The listing builds one solid part. Answer for the finished solid, in the listing's coordinates (mm). Face numbers are marked on the shaded views. A direction names the side the tool comes from. Round coordinates to 2 decimals unless told otherwise and drop trailing zeros. Loops run counter-clockwise (first coordinate to the right, second up) from the corner with the lowest first, then second, coordinate; pieces in that order, holes last. Notation, with made-up numbers: M 10,-25.75 L 29,-25.75 A23 ccw 29,-11.75 Z; hole C 6.5,17.5 d3. An arc over 180 degrees is marked long. Put each result on its own line as item: value. Start each with the question number.
(1) Which of the six approach directions +Z, -Z, +X, -X, +Y, -Y give full straight-line access (tool end or side, diameter ignored) to the marked faces 1, 2 and 3?
(2) Determine the mould class of the marked faces 4, 5, 6 and 7 for opening direction Z: released by +Z, released by -Z, zero draft, split by the parting line, or undercut.
(3) Section C-C, the plane y = 3.2 is taken. Determine the outline of the cut face in (x, z) (3 decimals).
(4) Straight lines are drawn through the part: line 1 (Y direction, x = -2.5, z = -3.25); line 2 (X direction, y = 1.45, z = -0.75); line 3 (Y direction, x = -1.25, z = 0.5). For each, find the intervals that lie inside material, in ascending order.
(5) Section D-D, the plane x = -2.75 is taken. Determine the outline of the cut face in (y, z), then the cut area to 3 significant figures.
(6) Flat-ended cylindrical pins translate along their axes: P1, Ø1, axis at y = 1.5, z = -2, coming from the +X side; P2, Ø1.5, axis at y = 3, z = -1, coming from the +X side; P3, Ø1.6, axis at x = -0.5, z = -0.5, coming from the -Y side. Find the tip coordinate at first contact, or state that the pin passes through.
(7) Section B-B, the plane x = -1 is taken. Determine the outline of the cut face in (y, z).
(8) Section A-A, the plane y = 0.3 is taken. Determine the outline of the cut face in (x, z) (3 decimals).
Autodesk Fusion 360 part; units mm, degrees
sketch "Sketch1" plane through (0, 0, 0) normal (0, 1, 0) x (1, 0, 0)
  line L0 (4.575, -1.7) -> (-4.575, -1.7)
  line L1 (-4.575, -1.7) -> (-4.575, 1.7)
  line L2 (-4.575, 1.7) -> (4.575, 1.7)
  line L3 (4.575, 1.7) -> (4.575, -1.7)
  line L4 (4.575, -1.7) -> (-4.575, 1.7) construction
  line L5 (-4.575, -1.7) -> (4.575, 1.7) construction
  dimension "d1" = 9.15
  dimension "d2" = 3.4
extrude "Extrude1" add sketch "Sketch1" along normal blind 4
sketch "Sketch2" plane through (0, 0, 0) normal (0, -1, 0) x (1, 0, 0)
  line L0 (-4.575, -1.7) -> (4.575, -1.7)
  line L1 (4.575, -1.7) -> (4.575, 1.7)
  line L2 (4.575, 1.7) -> (-4.575, 1.7)
  line L3 (-4.575, 1.7) -> (-4.575, -1.7)
  line L4 (6.575, -3.7) -> (-6.575, -3.7)
  line L5 (-6.575, -3.7) -> (-6.575, 3.7)
  line L6 (-6.575, 3.7) -> (6.575, 3.7)
  line L7 (6.575, 3.7) -> (6.575, -3.7)
  line L8 (6.575, -3.7) -> (-6.575, 3.7) construction
  line L9 (-6.575, -3.7) -> (6.575, 3.7) construction
  dimension "d5" = 13.15
  dimension "d6" = 7.4
extrude "Extrude2" add sketch "Sketch2" along normal blind 1 contours L0 L1 L2 L3 | L4 L5 L6 L7
fillet "Fillet1" radius 1.5 4 edges at (4.575, 2, 1.7) (4.575, 2, -1.7) (-4.575, 2, 1.7) (-4.575, 2, -1.7)
fillet "Fillet2" radius 0.5 8 edges at (4.1357, 4, -1.2607) (0, 4, -1.7) (-4.1357, 4, -1.2607) (-4.575, 4, 0) (-4.1357, 4, 1.2607) (0, 4, 1.7) (4.1357, 4, 1.2607) (4.575, 4, 0)
fillet "Fillet3" radius 1 4 edges at (6.575, -0.5, 3.7) (6.575, -0.5, -3.7) (-6.575, -0.5, 3.7) (-6.575, -0.5, -3.7)
sketch "Sketch3" plane through (0, -1, 0) normal (0, -1, 0) x (1, 0, 0)
  arc A0 (-6.575, -2.7) -> (-5.575, -3.7) centre (-5.575, -2.7) ccw
  line L0 (-5.575, -3.7) -> (5.575, -3.7)
  arc A1 (5.575, -3.7) -> (6.575, -2.7) centre (5.575, -2.7) ccw
  line L1 (6.575, -2.7) -> (6.575, 2.7)
  arc A2 (6.575, 2.7) -> (5.575, 3.7) centre (5.575, 2.7) ccw
  line L2 (5.575, 3.7) -> (-5.575, 3.7)
  arc A3 (-5.575, 3.7) -> (-6.575, 2.7) centre (-5.575, 2.7) ccw
  line L3 (-6.575, 2.7) -> (-6.575, -2.7)
  line L4 (1.6, -1.6) -> (-1.6, -1.6)
  line L5 (-1.6, -1.6) -> (-1.6, 1.6)
  line L6 (-1.6, 1.6) -> (1.6, 1.6)
  line L7 (1.6, 1.6) -> (1.6, -1.6)
  line L8 (1.6, -1.6) -> (-1.6, 1.6) construction
  line L9 (-1.6, -1.6) -> (1.6, 1.6) construction
  dimension "d12" = 3.2
  dimension "d13" = 3.2
extrude "Extrude3" cut sketch "Sketch3" against normal blind 2.7 contours L4 L5 L6 L7
chamfer "Chamfer1" distance 0.5 angle 45 4 edges at (1.6, -1, 0) (0, -1, -1.6) (0, -1, 1.6) (-1.6, -1, 0)
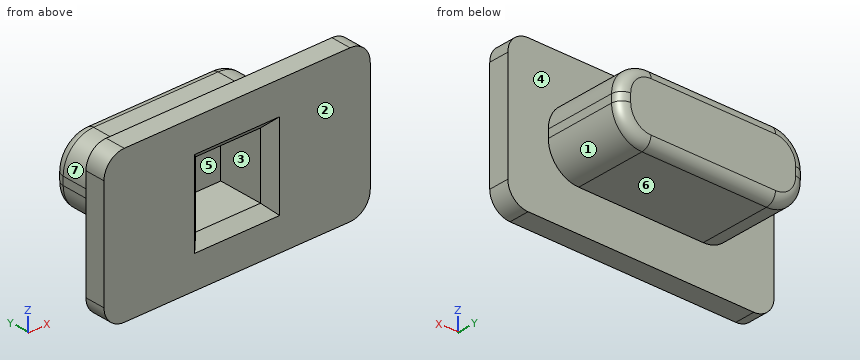
Recorded:
1. face 1: -Z, +X, +Y
1. face 2: +Z, -Z, +X, -X, -Y
1. face 3: -Y
2. face 4: zero draft
2. face 5: undercut
2. face 6: released by -Z
2. face 7: released by +Z
3. outline: M -4.575,-0.2 A1.5 ccw -3.075,-1.7 L 3.075,-1.7 A1.5 ccw 4.575,-0.2 L 4.575,0.2 A1.5 ccw 3.075,1.7 L -3.075,1.7 A1.5 ccw -4.575,0.2 Z
4. line 1: y = -1 to 0
4. line 2: x = -4.47 to -1.6, 1.6 to 4.47
4. line 3: y = 1.7 to 4
5. outline: M -1,-3.7 L 0,-3.7 L 0,-1.7 L 3.5,-1.7 A0.5 ccw 4,-1.2 L 4,1.2 A0.5 ccw 3.5,1.7 L 0,1.7 L 0,3.7 L -1,3.7 Z
5. area: 20.9 mm²
6. P1: stops at x = 3.82
6. P2: stops at x = 4.57
6. P3: stops at y = 1.7
7. outline: M -1,-3.7 L 0,-3.7 L 0,-1.7 L 3.5,-1.7 A0.5 ccw 4,-1.2 L 4,1.2 A0.5 ccw 3.5,1.7 L 0,1.7 L 0,3.7 L -1,3.7 L -1,2.1 L -0.5,1.6 L 1.7,1.6 L 1.7,-1.6 L -0.5,-1.6 L -1,-2.1 Z
8. outline: M -4.575,-0.2 A1.5 ccw -3.075,-1.7 L 3.075,-1.7 A1.5 ccw 4.575,-0.2 L 4.575,0.2 A1.5 ccw 3.075,1.7 L -3.075,1.7 A1.5 ccw -4.575,0.2 Z; hole M -1.6,-1.6 L 1.6,-1.6 L 1.6,1.6 L -1.6,1.6 Z
